from build123d import *

# Parameters (mm, degrees)
SKETCH1_W           = 127
SKETCH1_H           = 85
BOSS_EXTRUDE1_DEPTH = 10
CHAMFER1_SIZE       = 10
FILLET1_R           = 2
FILLET2_R           = 2
CUT_EXTRUDE1_DEPTH  = 7.3


with BuildPart() as part:
    # Sketch1 → Boss-Extrude1 (new body)
    with BuildSketch(Plane(origin=(0, 0, 0), x_dir=(1, 0, 0), z_dir=(0, 1, 0))):
        with Locations((63.5, -42.5)):
            Rectangle(SKETCH1_W, SKETCH1_H)
    extrude(amount=BOSS_EXTRUDE1_DEPTH)

    # Chamfer1
    chamfer1_edges = [part.edges().sort_by_distance(p)[0] for p in [
        (127, 5, 0),
        (127, 5, 85),
    ]]
    chamfer(chamfer1_edges, length=CHAMFER1_SIZE)

    # Fillet1
    fillet1_edges = [part.edges().sort_by_distance(p)[0] for p in [
        (127, 5, 10),
        (127, 5, 75),
        (117, 5, 85),
        (117, 5, 0),
        (0, 5, 0),
        (0, 5, 85),
    ]]
    fillet(fillet1_edges, radius=FILLET1_R)

    # Fillet2
    fillet2_edges = [part.edges().sort_by_distance(p)[0] for p in [
        (127, 10, 42.5),
        (122, 10, 80),
        (59.085786438, 10, 85),
        (122, 10, 5),
        (59.085786438, 10, 0),
        (0, 10, 42.5),
        (126.847759065, 10, 10.06306026),
        (116.93693974, 10, 0.152240935),
        (0.585786438, 10, 0.585786438),
        (0.585786438, 10, 84.414213562),
        (116.93693974, 10, 84.847759065),
        (126.847759065, 10, 74.93693974),
    ]]
    fillet(fillet2_edges, radius=FILLET2_R)

    # Sketch2 → Cut-Extrude1 (cut)
    with BuildSketch(Plane.XZ):
        Polygon((1.25, 83.75), (115.75, 83.75), (125.75, 73.75), (125.75, 11.25), (115.75, 1.25), (1.25, 1.25), align=None)
    extrude(amount=-CUT_EXTRUDE1_DEPTH, mode=Mode.SUBTRACT)


solid = part.part
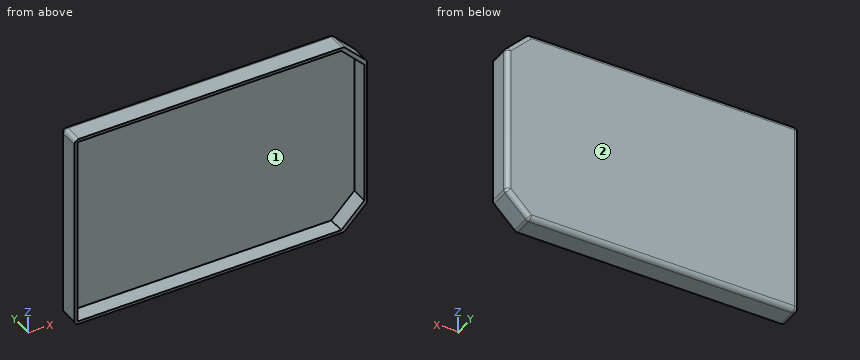
Geometry: final body of the model. Coordinates: model frame, mm. Face numbers are marked on the shaded views. Give positions to 0.01 mm unless a question says otherwise; leave off trailing zeros. Write each loop counter-clockwise with the first axis right and the second up, starting at its lowest first coordinate (ties: lowest second). Pieces come first, ordered by that corner, then holes. Notation, with made-up numbers: (18.5, 6.5) -> (58.5, 6.5) arc R20 cw to (58.5, 37.5) -> close; hole circle Ø8 at (-20, -20.5). An arc over 180 degrees is marked (long way). Answer as a JSON object with one key per item and string values.
1. Mould query, pull axis Z, two halves, no side actions, for the marked faces 1 and 2. Classes: pulls with the +Z half, pulls with the -Z half, needs draft (parallel to the pull), parting line crosses it, or undercut.
Ans:
{"face 1": "undercut", "face 2": "needs draft"}
2. Cut plane B-B on z = 50. Output: boundary loops of the cut face in (x, y).
Ans:
{"outline": "(0, 0) -> (1.25, 0) -> (1.25, 7.3) -> (125.75, 7.3) -> (125.75, 0) -> (127, 0) -> (127, 8) arc R2 ccw to (125, 10) -> (2, 10) arc R2 ccw to (0, 8) -> close"}
3. Contact query for a flat-ended pin moving along its axis: pin 1 (3 mm diameter, centred on x = 111, z = 59.5, fed in from -Y). Output: stop coordinate, or through.
Ans:
{"pin 1": "stops at y = 7.3"}
4. Cut plane A-A on y = 4.75. Output: boundary loops of the cut face in (x, z), and give its area (3 significant figures).
Ans:
{"outline": "(0, 2) arc R2 ccw to (2, 0) -> (116.17, 0) arc R2 ccw to (117.59, 0.59) -> (126.41, 9.41) arc R2 ccw to (127, 10.83) -> (127, 74.17) arc R2 ccw to (126.41, 75.59) -> (117.59, 84.41) arc R2 ccw to (116.17, 85) -> (2, 85) arc R2 ccw to (0, 83) -> close; hole (1.25, 1.25) -> (115.75, 1.25) -> (125.75, 11.25) -> (125.75, 73.75) -> (115.75, 83.75) -> (1.25, 83.75) -> close", "area": "522 mm^2"}
5. Ray query, probe 1 along Z at (x, y) = (41, 1.75); probe 2 along X at (y, z) = (6.5, 33.5); probe 3 along Y at (x, z) = (104, 42.5). Return the intervals inside material, ascending. Write a range as from..to.
Ans:
{"probe 1": "z = 0..1.25, 83.75..85", "probe 2": "x = 0..1.25, 125.75..127", "probe 3": "y = 7.3..10"}
6. Cut plane C-C on x = 111.5. Output: boundary loops of the cut face in (y, z).
Ans:
{"outline": "(0, 0) -> (8, 0) arc R2 ccw to (10, 2) -> (10, 83) arc R2 ccw to (8, 85) -> (0, 85) -> (0, 83.75) -> (7.3, 83.75) -> (7.3, 1.25) -> (0, 1.25) -> close"}
